Autodesk Inventor part; units mm, degrees
ref_plane "YZ Plane" through (0, 0, 0) normal (1, 0, 0) x (0, 1, 0)
ref_plane "XY Plane" through (0, 0, 0) normal (0, 0, 1) x (1, 0, 0)
sketch "スケッチ1" plane through (0, 0, 0) normal (1, 0, 0) x (0, 1, 0)
  arc A0 (-2.7792, 1.1297) -> (2.7792, -1.1297) centre (0, 0) ccw
  circle A1 centre (5, 12.3) radius 1.7
  arc A2 (7.7792, 11.1703) -> (2.2208, 13.4297) centre (5, 12.3) ccw
  circle A3 centre (0, 0) radius 1.7
  line L0 (2.2208, 13.4297) -> (-2.7792, 1.1297)
  line L1 (7.7792, 11.1703) -> (2.7792, -1.1297)
  dimension "d1" = 3.4
  dimension "d2" = 6
  dimension "d3" = 3.4
  dimension "d4" = 5
  dimension "d5" = 12.3
  dimension "d8" = 3
extrude "押し出し1" add sketch "スケッチ1" against normal blind 6.2
sketch "スケッチ2" plane through (0, 0, 0) normal (1, 0, 0) x (0, 0, -1)
  circle A0 centre (0, 0) radius 1.7
  circle A1 centre (-12.3, 5) radius 1.7
  line L0 (-1.1297, -2.7792) -> (-13.4297, 2.2208)
  arc A2 (-1.1297, -2.7792) -> (1.1297, 2.7792) centre (0, 0) ccw
  line L1 (-11.1703, 7.7792) -> (1.1297, 2.7792)
  arc A3 (-11.1703, 7.7792) -> (-13.4297, 2.2208) centre (-12.3, 5) ccw
  circle A4 centre (0, 0) radius 3
  line L2 (-1.1297, -2.7792) -> (1.1297, 2.7792)
  dimension "d11" = 6
extrude "押し出し2" cut sketch "スケッチ2" against normal blind 1.7 contours A4 L0 A3 L1
sketch "スケッチ3" plane through (-6.2, 0, 0) normal (-1, 0, 0) x (0, 0, 1)
  circle A0 centre (0, 0) radius 1.7
  circle A1 centre (12.3, 5) radius 1.7
  line L0 (1.1297, -2.7792) -> (13.4297, 2.2208)
  arc A2 (13.4297, 2.2208) -> (11.1703, 7.7792) centre (12.3, 5) ccw
  line L1 (11.1703, 7.7792) -> (-1.1297, 2.7792)
  arc A3 (-1.1297, 2.7792) -> (1.1297, -2.7792) centre (0, 0) ccw
  circle A4 centre (12.3, 5) radius 3
  line L2 (11.1703, 7.7792) -> (13.4297, 2.2208)
  line L3 (1.1297, -2.7792) -> (13.4297, 2.2208)
  dimension "d14" = 6
extrude "押し出し3" cut sketch "スケッチ3" against normal blind 1.7 contours A4 L0 A3 L1
sketch "スケッチ4" plane through (-1.7, 0, 0) normal (1, 0, 0) x (0, 0, -1)
  arc A0 (1.1297, 2.7792) -> (-1.1297, -2.7792) centre (0, 0) ccw
  line L0 (-11.1703, 7.7792) -> (1.1297, 2.7792)
  arc A1 (-11.1703, 7.7792) -> (-13.4297, 2.2208) centre (-12.3, 5) ccw
  line L1 (-1.1297, -2.7792) -> (-13.4297, 2.2208)
  circle A2 centre (-12.3, 5) radius 1.7
  line L2 (-13.4297, 2.2208) -> (-13.8977, 1.0697)
  line L3 (-13.8977, 1.0697) -> (-15.064, 3.8337)
  arc A3 (-11.1703, 7.7792) -> (-13.4297, 2.2208) centre (-12.3, 5) ccw
  dimension "d17" = 45
extrude "押し出し4" add sketch "スケッチ4" against normal up to surface (4.5 mm away) contours L2 L3 A1
mirror "ミラー1" about plane through (-1.7, 2.2208, 13.4297) normal (0, -0.3765791, -0.9263845) of "押し出し4"
sketch "スケッチ5" plane through (-1.7, 0, 0) normal (1, 0, 0) x (0, 0, -1)
  line L0 (-1.1297, -2.7792) -> (-12.2786, 1.7529)
  arc A0 (1.1297, 2.7792) -> (-1.1297, -2.7792) centre (0, 0) ccw
  line L1 (-11.1703, 7.7792) -> (1.1297, 2.7792)
  arc A1 (-11.1703, 7.7792) -> (-15.064, 3.8337) centre (-12.3, 5) ccw
  line L2 (-15.064, 3.8337) -> (-13.8977, 1.0697)
  line L3 (-12.2786, 1.7529) -> (-13.8977, 1.0697)
  circle A2 centre (-12.3, 5) radius 1.7
  line L4 (-12.9402, 3.4251) -> (-13.2054, 2.7728)
  line L5 (-13.2054, 2.7728) -> (-13.8663, 4.3391)
  circle A3 centre (-12.3, 5) radius 1.7
  arc A4 (-13.8663, 4.3391) -> (-12.9402, 3.4251) centre (-12.3, 5) ccw
  dimension "d20" = 45
extrude "押し出し5" cut sketch "スケッチ5" against normal blind 10 contours A2 L4 L5
mirror "ミラー2" about plane through (-1.7, 3.4251, 12.9402) normal (0, 0.3765791, 0.9263845) of "押し出し5"
fillet "フィレット1" radius 1.3 1 edges at (-3.95, 1.0697, 13.8977)
sketch "スケッチ6" plane through (-4.5, 0, 0) normal (-1, 0, 0) x (0, 0, 1)
  circle A0 centre (0, 0) radius 1.7
  line L0 (12.2786, 1.7529) -> (11.1337, 2.236)
  arc A1 (11.1703, 7.7792) -> (11.1337, 2.236) centre (12.3, 5) ccw
  line L1 (-1.1297, 2.7792) -> (11.1703, 7.7792)
  arc A2 (-1.1297, 2.7792) -> (1.1297, -2.7792) centre (0, 0) ccw
  line L2 (12.2786, 1.7529) -> (1.1297, -2.7792)
  line L3 (1.1297, -2.7792) -> (1.5977, -3.9303)
  line L4 (1.5977, -3.9303) -> (-1.1663, -2.764)
  dimension "d24" = 45
extrude "押し出し6" add sketch "スケッチ6" against normal up to surface (4.5 mm away) contours L3 L4 A2
mirror "ミラー3" about plane through (-4.5, -2.7792, 1.1297) normal (0, 0.3765791, 0.9263845) of "押し出し6"
sketch "スケッチ7" plane through (-4.5, 0, 0) normal (-1, 0, 0) x (0, 0, 1)
  circle A0 centre (0, 0) radius 1.7
  line L0 (0.6402, -1.5749) -> (0.9054, -2.2272)
  line L1 (0.9054, -2.2272) -> (-0.6609, -1.5663)
  line L2 (-1.1297, 2.7792) -> (11.1703, 7.7792)
  dimension "d29" = 45
extrude "押し出し7" cut sketch "スケッチ7" against normal blind 10 contours A0 L0 L1
mirror "ミラー4" about plane through (-4.5, -1.5749, 0.6402) normal (0, -0.3765791, -0.9263845) of "押し出し7"
fillet "フィレット2" radius 1.3 1 edges at (-2.25, -3.9303, 1.5977)
sketch "スケッチ8" plane through (-4.5, 0, 0) normal (-1, 0, 0) x (0, 0, 1)
  line L0 (-1.1297, 2.7792) -> (11.1703, 7.7792)
  arc A0 (-1.1297, 2.7792) -> (-1.1663, -2.764) centre (0, 0) ccw
  line L1 (-1.1297, 2.7792) -> (-2.7291, 2.129)
  line L2 (-2.7291, 2.129) -> (-2.9705, 0.4196)
extrude "押し出し8" add sketch "スケッチ8" against normal up to surface (4.5 mm away)
ref_plane "作業平面1" through (0, 2.7792, -1.1297) normal (0, -0.3765791, -0.9263845) x (-1, 0, 0)
mirror "ミラー5" about plane through (0, 2.7792, -1.1297) normal (0, -0.3765791, -0.9263845) of "押し出し8"
sketch "スケッチ9" plane through (-6.2, 0, 0) normal (-1, 0, 0) x (0, 0, 1)
  arc A0 (12.7, 1.5751) -> (14.4031, 2.2674) centre (13.2054, 2.7728) ccw
  line L0 (14.4031, 2.2674) -> (15.064, 3.8337)
  arc A1 (15.064, 3.8337) -> (11.1337, 2.236) centre (12.3, 5) ccw
  line L1 (12.7, 1.5751) -> (11.1337, 2.236)
  line L2 (13.2054, 2.7728) -> (11.6391, 3.4337)
  arc A2 (13.8663, 4.3391) -> (11.6391, 3.4337) centre (12.3, 5) ccw
  line L3 (13.8663, 4.3391) -> (13.2054, 2.7728)
  line L4 (-2.7291, 2.129) -> (11.1703, 7.7792)
  line L5 (11.1703, 7.7792) -> (12.4648, 8.3054)
  line L6 (12.4648, 8.3054) -> (13.7006, 7.653)
  point P0 (0, 0)
extrude "押し出し9" add sketch "スケッチ9" against normal up to surface (4.5 mm away) contours L5 L6 A1
ref_plane "作業平面2" through (0, 7.7792, 11.1703) normal (0, -0.3765791, -0.9263845) x (-1, 0, 0)
mirror "ミラー6" about plane through (0, 7.7792, 11.1703) normal (0, -0.3765791, -0.9263845) of "押し出し9"
ref_plane "作業平面3" through (0, 7.7792, 11.1703) normal (0, -0.3765791, -0.9263845) x (-1, 0, 0)
scale "尺度1" factors (0.8836555, 0.8836555, 0.8836555) then translate (-0.5236, -0.0325, 0.847) bodies 1
properties part number "HbRing-LittleCouplerLink01" material "ナイロン 6/6"
Verification items for the finished model (mm, model axes). A direction names the side the tool comes from. Give positions to 0.01 mm unless a question says otherwise; leave off trailing zeros. Order: outer loops, then holes, each group sorted by start corner. A loop starts at its lowest first (then second) coordinate and runs counter-clockwise, first axis right, second up. Notation, with made-up numbers: (15, 71.5) -> (23, 71.5) arc R22 ccw to (23, 105.5) -> close; hole circle Ø11 at (30.5, 77). An arc over 180 degrees is marked (long way). Use a Markdown table: item, result.
1) Tool access check on faces 1 (the flat face through (-4.9, 1.6, 11.5)), 2 (the cylindrical face through (-5.262, 3.307, 9.294)), 3 (the flat face through (-2.54, -1.71, 0.96)), 4 (the flat face through (-1.656, -1.899, 2.937)). Record the directions out of +Z, -Z, +X, -X, +Y, -Y that give a thin tool (end or side, any length) a straight path to the whole face; none if there is none.
Results:
| item | result |
|---|---|
| face 1 | -X, -Y |
| face 2 | -Z, -X |
| face 3 | +X, -X |
| face 4 | +Z, +X, -Y |
2) Section check D-D, the plane x = -2.5. Record the boundary of the cut face in (y, z), then the cut area to 3 significant figures.
Results:
| item | result |
|---|---|
| outline | (-3.06, 1.2) -> (-2.47, -0.18) arc R2.65 ccw to (0.34, -1.78) -> (1.85, -1.56) -> (2.42, -0.15) -> (6.84, 10.72) -> (7.31, 11.86) -> (6.73, 12.95) arc R2.65 ccw to (3.36, 14.16) -> (1.97, 13.57) arc R1.15 ccw to (1.36, 12.07) -> (1.52, 11.7) -> (-2.07, 2.86) -> (-2.45, 2.71) arc R1.15 ccw to start; hole (-2, 1.65) -> (-1.42, 0.26) arc R1.5 ccw (long way) to (-0.62, 2.23) -> close; hole (2.42, 12.52) -> (3, 11.13) arc R1.5 ccw (long way) to (3.8, 13.1) -> close |
| area | 71.9 mm² |
3) Section check C-C, the plane x = -1.2. Record the boundary of the cut face in (y, z).
Results:
| item | result |
|---|---|
| outline | (-3.06, 1.2) -> (-2.47, -0.18) arc R2.65 ccw to (0.34, -1.78) -> (1.85, -1.56) -> (2.42, -0.15) -> (3, 1.26) -> (2.06, 2.47) arc R2.65 ccw to (-1.06, 3.29) -> (-2.45, 2.71) arc R1.15 ccw to start; hole (-2, 1.65) -> (-1.42, 0.26) arc R1.5 ccw (long way) to (-0.62, 2.23) -> close |
4) Depth check by flat-ended pin: pin 1 Ø4.5 at (y, z) = (0.5, 6.5) entering from +X; pin 2 Ø5 at (y, z) = (1, 3.5) entering from +X; pin 3 Ø6 at (y, z) = (4.5, 3) entering from -X; pin 4 Ø1.5 at (x, z) = (-2, 8) entering from +Y. Enter the tip coordinate at first touch or a pass-through.
Results:
| item | result |
|---|---|
| pin 1 | x = -2.03 |
| pin 2 | x = -0.52 |
| pin 3 | x = -4.5 |
| pin 4 | y = 6.04 |
5) Material ranges on probe 1 along X at (y, z) = (-1.25, -0.5); probe 2 along X at (y, z) = (5.5, 8.25); probe 3 along Y at (x, z) = (-1, 0.75), recorded low to high.
Results:
| item | result |
|---|---|
| probe 1 | -4.5 to -0.52 |
| probe 2 | -4.5 to -2.03 |
| probe 3 | -2.87 to -1.62, 1.47 to 2.79 |
6) Section check A-A, the plane y = 1. Record the boundary of the cut face in (x, z), then the cut area to 3 significant figures.
Results:
| item | result |
|---|---|
| outline | (-4.5, -1.68) -> (-0.52, -1.68) -> (-0.52, -0.24) -> (-4.5, -0.24) -> close; (-4.5, 1.94) -> (-0.52, 1.94) -> (-0.52, 3.29) -> (-2.03, 3.29) -> (-2.03, 10.43) -> (-4.5, 10.43) -> close |
| area | 28.8 mm² |
7) Section check B-B, the plane z = 1. Record the boundary of the cut face in (x, y).
Results:
| item | result |
|---|---|
| outline | (-4.5, -2.97) -> (-0.52, -2.97) -> (-0.52, -1.73) -> (-4.5, -1.73) -> close; (-4.5, 1.46) -> (-0.52, 1.46) -> (-0.52, 2.89) -> (-4.5, 2.89) -> close |
8) Mould release check, pull along Y, two halves, no side actions. Record for faces 5 (the flat face through (-0.524, 1, -1)), 6 (the cylindrical face through (-3.986, 5.758, 11.105)), 7 (the cylindrical face through (-2.48, -3.06, 2.09)): pulls with the +Y half, pulls with the -Y half, needs draft (parallel to the pull), parting line crosses it, or undercut.
Results:
| item | result |
|---|---|
| face 5 | needs draft |
| face 6 | undercut |
| face 7 | pulls with the -Y half |
